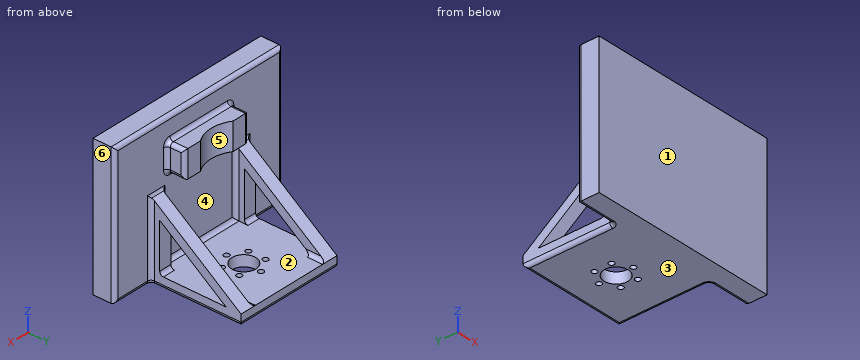
from build123d import *

# Parameters (mm, degrees)
BOSS_EXTRUDE1_DEPTH = 52.5
SKETCH6_W           = 40
SKETCH6_H           = 15
BOSS_EXTRUDE3_DEPTH = 10
SKETCH9_R           = 6.65
SKETCH9_R_2         = 1.5
CUT_EXTRUDE4_DEPTH  = 78
CIRPATTERN2_COUNT   = 6
SKETCH10_R          = 18.125
CUT_EXTRUDE5_DEPTH  = 72
FILLET3_R           = 2
SKETCH11_W          = 22.5
SKETCH11_H          = 50
CUT_EXTRUDE6_DEPTH  = 7
BOSS_EXTRUDE4_DEPTH = 7
CUT_EXTRUDE8_DEPTH  = 83.5
FILLET5_R           = 2


with BuildPart() as part:
    # Sketch1 → Boss-Extrude1 (new body, symmetric)
    with BuildSketch(Plane(origin=(0, 0, 0), x_dir=(0, 0, -1), z_dir=(1, 0, 0))):
        Polygon((0, 0), (0, 50), (6, 50), (6, -12), (-71, -12), (-71, 0), align=None)
    extrude(amount=BOSS_EXTRUDE1_DEPTH, both=True)

    # Sketch6 → Boss-Extrude3 (add)
    with BuildSketch(Plane(origin=(0, 0, 0), x_dir=(1, 0, 0), z_dir=(0, 1, 0))):
        with Locations((0, -51.25)):
            Rectangle(SKETCH6_W, SKETCH6_H)
    extrude(amount=BOSS_EXTRUDE3_DEPTH)

    # Sketch9 → Cut-Extrude4 (cut, through all)
    with BuildSketch(Plane(origin=(0, 0, -6), x_dir=(-1, 0, 0), z_dir=(0, 0, -1))):
        with Locations((0, 25)):
            Circle(SKETCH9_R)
        with Locations((0, 34.5)):
            Circle(SKETCH9_R_2)
    cut_extrude4 = extrude(amount=-CUT_EXTRUDE4_DEPTH, mode=Mode.SUBTRACT)

    # CirPattern2: Cut-Extrude4 ×6 about axis
    cirpattern2_axis = Axis((0, 25, 0), (0, 0, 1))
    for i in range(1, CIRPATTERN2_COUNT):
        add(cut_extrude4.rotate(cirpattern2_axis, i * 360 / CIRPATTERN2_COUNT), mode=Mode.SUBTRACT)

    # Sketch10 → Cut-Extrude5 (cut, through all)
    with BuildSketch(Plane.XY):
        with Locations((0, 25)):
            Circle(SKETCH10_R)
    extrude(amount=CUT_EXTRUDE5_DEPTH, mode=Mode.SUBTRACT)

    # Fillet3
    fillet3_edges = [part.edges().sort_by_distance(p)[0] for p in [
        (-20, 0, 51.25),
        (-20, 5, 43.75),
        (0, 0, 58.75),
        (-20, 5, 58.75),
        (20, 0, 51.25),
        (20, 5, 58.75),
        (0, 0, 43.75),
        (20, 5, 43.75),
        (-20, 10, 51.25),
        (20, 10, 51.25),
    ]]
    fillet(fillet3_edges, radius=FILLET3_R)

    # Sketch11 → Cut-Extrude6 (cut, through all)
    with BuildSketch(Plane.XY):
        with Locations((-41.25, 25)):
            Rectangle(SKETCH11_W, SKETCH11_H)
    cut_extrude6 = extrude(amount=-CUT_EXTRUDE6_DEPTH, mode=Mode.SUBTRACT)

    # Mirror1: Cut-Extrude6 across plane
    add(cut_extrude6.mirror(Plane(origin=(0, 0, 0), x_dir=(0, 0, 1), z_dir=(1, 0, 0))), mode=Mode.SUBTRACT)

    # Sketch13 → Boss-Extrude4 (add)
    with BuildSketch(Plane(origin=(30, 0, 0), x_dir=(0, 0, -1), z_dir=(1, 0, 0))):
        Polygon((0, 0), (-36.962201233, 0), (0, 50), align=None)
    boss_extrude4 = extrude(amount=-BOSS_EXTRUDE4_DEPTH)

    # Sketch14 → Cut-Extrude8 (cut, through all)
    with BuildSketch(Plane(origin=(30, 0, 0), x_dir=(0, 0, -1), z_dir=(1, 0, 0))):
        Polygon((-27.048100185, 5), (0, 5), (0, 41.588865493), align=None)
    cut_extrude8 = extrude(amount=-CUT_EXTRUDE8_DEPTH, mode=Mode.SUBTRACT)

    # Mirror2: Boss-Extrude4, Cut-Extrude8 across plane
    add(boss_extrude4.mirror(Plane(origin=(0, 0, 0), x_dir=(0, 0, 1), z_dir=(1, 0, 0))))
    add(cut_extrude8.mirror(Plane(origin=(0, 0, 0), x_dir=(0, 0, 1), z_dir=(1, 0, 0))), mode=Mode.SUBTRACT)

    # Fillet5
    fillet5_edges = [part.edges().sort_by_distance(p)[0] for p in [
        (30, 25, -6),
        (-30, 25, -6),
        (23, 0, 18.481100617),
        (26.5, 0, 36.962201233),
        (30, 0, 15.481100617),
        (41.25, 0, -6),
        (52.5, 0, 32.5),
        (0, 0, 71),
        (-52.5, 0, 32.5),
        (-41.25, 0, -6),
        (-30, 0, 15.481100617),
        (-26.5, 0, 36.962201233),
        (-23, 0, 18.481100617),
        (0, 0, 0),
        (0, 50, -6),
        (23, 45.794432746, 0),
        (-23, 45.794432746, 0),
        (26.5, 5, 0),
        (-26.5, 5, 0),
    ]]
    fillet(fillet5_edges, radius=FILLET5_R)


solid = part.part
Geometry: final body of the model. Coordinates: model frame, mm. Face numbers are marked on the shaded views. A direction names the side the tool comes from. Round coordinates to 2 decimals unless told otherwise and drop trailing zeros. Loops run counter-clockwise (first coordinate to the right, second up) from the corner with the lowest first, then second, coordinate; pieces in that order, holes last. Notation, with made-up numbers: M 16.25,-38 L 54.25,-38 A17 cw 54.25,-10 Z; hole C 27,88.25 d5. An arc over 180 degrees is marked long. One line per question, with ' | ' between items.
(1) Contact query for flat-ended pins moving along their axis: P1, Ø17.5, axis at y = 20, z = 24, coming from the +X side; P2, Ø6.5, axis at y = 4.5, z = 50.5, coming from the +X side; P3, Ø15.5, axis at x = 0, y = 25, coming from the +Z side; P4, Ø2.5, axis at x = 8.23, y = 29.75, coming from the -Z side. Output: stop coordinate, or through.
Check result:
P1: stops at x = 30 | P2: stops at x = 20.15 | P3: stops at z = 0 | P4: passes through
(2) Cut plane B-B on y = 15.5. Return the cut outline in (x, z).
Check result:
outline: M -30,-4 A2 ccw -28,-6 L -1.5,-6 L -1.5,0 L -30,0 Z; M -30,19.29 L -23,19.29 L -23,25.5 L -30,25.5 Z; M 1.5,-6 L 28,-6 A2 ccw 30,-4 L 30,0 L 1.5,0 Z; M 23,19.29 L 30,19.29 L 30,25.5 L 23,25.5 Z
(3) Access query for the marked faces 5 and 6. Directions: +Z, -Z, +X, -X, +Y, -Y. A direction counts if a zero-diameter tool reaches every point of the face in a straight line with its end or side. Return the directions, or none.
Check result:
face 5: +Z, +Y | face 6: +Z, -Z, +X, +Y, -Y
(4) Cut plane C-C on z = 51. Return the cut outline in (x, y) (3 decimals), plus the area to 3 significant figures.
Check result:
outline: M -52.5,-12 L 52.5,-12 L 52.5,-2 A2 ccw 50.5,0 L 22,0 A2 cw 20,2 L 20,8 A2 ccw 18,10 L 10.174,10 A18.125 cw -10.174,10 L -18,10 A2 ccw -20,8 L -20,2 A2 cw -22,0 L -50.5,0 A2 ccw -52.5,-2 Z | area: 1,620 mm2
(5) Pull-direction query (Z, two-part tool) for the marked faces 1, 2, 3 and 4; classes: +Z half, -Z half, draft (parallel to the pull), parting line (faces both ways), or undercut.
Check result:
face 1: draft | face 2: undercut | face 3: -Z half | face 4: undercut
(6) Material intervals for line 1 along Y through (x, z) = (0, -1.25); line 2 along X through (y, z) = (29, -1); line 3 along Y through (x, z) = (-40, 14.5), sorted ascending. Write a range as from..to.
Check result:
line 1: y = -12..14, 17..18.35, 31.65..33, 36..50 | line 2: x = -30..-9.53, -6.93..-5.31, 5.31..6.93, 9.53..30 | line 3: y = -12..0
(7) Cut plane D-D on z = 10. Return the cut outline in (x, y), plus the area to 3 significant figures.
Check result:
outline: M -52.5,-12 L 52.5,-12 L 52.5,-2 A2 ccw 50.5,0 L 32,0 A2 cw 30,2 L 30,5 L 23,5 L 23,2 A2 cw 21,0 L -21,0 A2 cw -23,2 L -23,5 L -30,5 L -30,2 A2 cw -32,0 L -50.5,0 A2 ccw -52.5,-2 Z; M -30,28.06 L -23,28.06 L -23,36.47 L -30,36.47 Z; M 23,28.06 L 30,28.06 L 30,36.47 L 23,36.47 Z | area: 1,450 mm2
(8) Cut plane A-A on x = 0. Return the cut outline in (y, z) (3 decimals).
Check result:
outline: M -12,-6 L 14,-6 L 14,0 L 2,0 A2 cw 0,2 L 0,41.75 A2 cw 2,43.75 L 6.875,43.75 L 6.875,58.75 L 2,58.75 A2 cw 0,60.75 L 0,69 A2 ccw -2,71 L -12,71 Z; M 17,-6 L 18.35,-6 L 18.35,0 L 17,0 Z; M 31.65,-6 L 33,-6 L 33,0 L 31.65,0 Z; M 36,-6 L 48,-6 A2 ccw 50,-4 L 50,0 L 36,0 Z
